Geometry: final body of the model. Coordinates: model frame, mm. A direction names the side the tool comes from. Coordinates: 2 decimals unless noted, no trailing zeros. One line per item, written item: value.
```python
from build123d import *

# Parameters (mm, degrees)
BOSS_EXTRUDE1_DEPTH = 20
CUT_EXTRUDE1_START  = -5
SKETCH2_W           = 40
SKETCH2_H           = 16
CUT_EXTRUDE1_DEPTH  = 62.708320486


with BuildPart() as part:
    # Sketch1 → Boss-Extrude1 (new body)
    with BuildSketch(Plane.XY):
        with BuildLine():
            Line((0, 0), (0, 45))
            add(Edge.make_bspline(
                [(0, 45), (-6.04309054, 34.377032995), (-19.596555361, 18.290474097), (-36.768954214, 5.047598121), (-45, 0)],
                knots=[0, 0, 0, 0, 0.55, 1, 1, 1, 1], degree=3))
            Line((-45, 0), (0, 0))
        make_face()
    extrude(amount=BOSS_EXTRUDE1_DEPTH)

    # Sketch2 → Cut-Extrude1 (cut, through all)
    with BuildSketch(Plane.XZ.offset(CUT_EXTRUDE1_START)):
        with Locations((-25, 10)):
            Rectangle(SKETCH2_W, SKETCH2_H)
    extrude(amount=-CUT_EXTRUDE1_DEPTH, mode=Mode.SUBTRACT)


solid = part.part
```
(1) Reachability of faces 5 (the flat face through (-23, 0, 10)), 6 (the flat face through (-21, 5, 10)) from +Z, -Z, +X, -X, +Y, -Y: full face, straight path, thin tool, end or side. Return the list, or none.
Responses:
face 5: +Z, -Z, +X, -X, -Y
face 6: -X, +Y
(2) Line query: line 1 (Z direction, x = -25, y = 10.5); line 2 (Y direction, x = -31.5, z = 16); line 3 (X direction, y = 36.5, z = 9). Output: solid intervals per line, ascending. Write a range as [from, to].
Responses:
line 1: z = [0, 2], [18, 20]
line 2: y = [0, 5]
line 3: x = [-5, 0]
(3) Pull-direction query (Z, two-part tool) for faces 1 (the flat face through (0, 22, 10)), 2 (the flat face through (-13, 13, 20)), 3 (the flat face through (-13, 13, 0)), 4 (the flat face through (-14, 14, 18)); classes: released by +Z, released by -Z, zero draft, split by the parting line, or undercut.
Responses:
face 1: zero draft
face 2: released by +Z
face 3: released by -Z
face 4: undercut
(4) First-contact query: pin 1 (3 mm diameter, centred on x = -34.5, z = 4.5, fed in from +Y); pin 2 (5 mm diameter, centred on x = -34, y = 12, fed in from -Z); pin 3 (1.5 mm diameter, centred on y = 37.5, z = 6.5, fed in from -X). Flat tips, straight axial feed; report the tip coordinate or a pass-through.
Responses:
pin 1: stops at y = 5
pin 2: passes through
pin 3: stops at x = -5
